For this review, use the dimensioned drawing (mm, ordinates from the lowest corner) and the shaded views. Round coordinates to 2 decimals unless told otherwise and drop trailing zeros. Write each loop counter-clockwise with the first axis right and the second up, starting at its lowest first coordinate (ties: lowest second). Pieces come first, ordered by that corner, then holes. Notation, with made-up numbers: M 26.5,63 L 48.5,63 A25 ccw 48.5,92 Z; hole C -28.5,9.5 d5. An arc over 180 degrees is marked long. One line per question, with ' | ' between items. Start each with the question number.
Item 1: For L1, parallel to Y at x = 120, z = 3.5; L2, parallel to Z at x = 62, y = 2.75; L3, parallel to Y at x = 48.5, z = 2.25, list the stretches that pass through material, from the lowest coordinate up.
Item 2: Add section A-A, the plane z = 5.25. State the section outline as (x, y) points.
Item 3: Insertion check: pin 1 Ø1.5 at (x, y) = (34.5, 1.5) entering from +Z; pin 2 Ø1.5 at (x, z) = (124, 5) entering from -Y. Each pin has a flat end and moves straight along its axis. Give the tip position at first contact, or say it passes through.
Item 4: Add section C-C, the plane x = 65. State the section outline as (y, z) points (3 decimals).
Item 5: Add section B-B, the plane y = 4.5. State the section outline as (x, z) points, and give its area (3 significant figures).
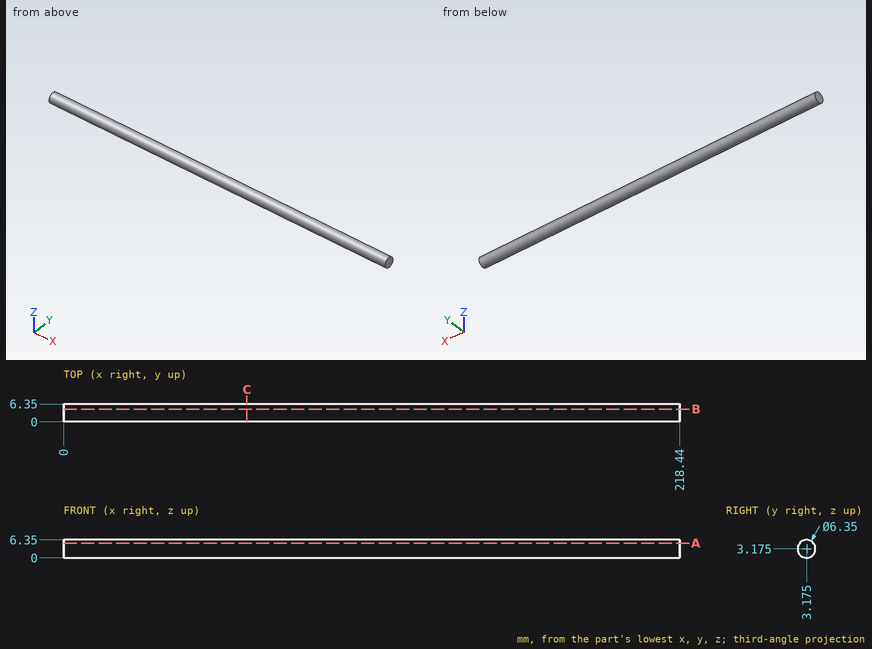
Computed values:
1) L1: y = 0.02 to 6.33 | L2: z = 0.03 to 6.32 | L3: y = 0.14 to 6.21
2) outline: M 0,0.77 L 218.44,0.77 L 218.44,5.58 L 0,5.58 Z
3) pin 1: stops at z = 6.21 | pin 2: stops at y = 0.19
4) outline: C 3.175,3.175 d6.35
5) outline: M 0,0.29 L 218.44,0.29 L 218.44,6.06 L 0,6.06 Z | area: 1,260 mm^2
